```python
from build123d import *

# Parameters (mm, degrees)
SKETCH_1_R      = 1.6
EXTRUDE_1_DEPTH = 2
FILLET_1_R      = 2


with BuildPart() as part:
    # 草图1 → 凸台-拉伸1 (new body)
    with BuildSketch(Plane(origin=(0, 0, 0), x_dir=(1, 0, 0), z_dir=(0, 1, 0))):
        with BuildLine():
            Line((-130, -81.5), (130, -81.5))
            Line((130, -81.5), (130, 81.5))
            Line((130, 81.5), (90, 81.5))
            ThreePointArc((90, 81.5), (0, -8.5), (-90, 81.5))
            Line((-90, 81.5), (-130, 81.5))
            Line((-130, 81.5), (-130, -81.5))
        make_face()
        with Locations(Location((-122, -33.5, 0), (0, 0, 270))):
            Circle(SKETCH_1_R, mode=Mode.SUBTRACT)
        with Locations(Location((-122, -13.5, 0), (0, 0, 270))):
            Circle(SKETCH_1_R, mode=Mode.SUBTRACT)
        with Locations(Location((-122, 36.5, 0), (0, 0, 270))):
            Circle(SKETCH_1_R, mode=Mode.SUBTRACT)
        with Locations(Location((-82.27241336, 34, 0), (0, 0, 270))):
            Circle(SKETCH_1_R, mode=Mode.SUBTRACT)
        with Locations(Location((-47.5, -0.77241336, 0), (0, 0, 270))):
            Circle(SKETCH_1_R, mode=Mode.SUBTRACT)
        with Locations(Location((122, -33.5, 0), (0, 0, 270))):
            Circle(SKETCH_1_R, mode=Mode.SUBTRACT)
        with Locations(Location((0, -13.5, 0), (0, 0, 270))):
            Circle(SKETCH_1_R, mode=Mode.SUBTRACT)
        with Locations(Location((47.5, -0.77241336, 0), (0, 0, 270))):
            Circle(SKETCH_1_R, mode=Mode.SUBTRACT)
        with Locations(Location((122, -13.5, 0), (0, 0, 270))):
            Circle(SKETCH_1_R, mode=Mode.SUBTRACT)
        with Locations(Location((82.27241336, 34, 0), (0, 0, 270))):
            Circle(SKETCH_1_R, mode=Mode.SUBTRACT)
        with Locations(Location((122, 36.5, 0), (0, 0, 270))):
            Circle(SKETCH_1_R, mode=Mode.SUBTRACT)
        with Locations(Location((-122, 56.5, 0), (0, 0, 270))):
            Circle(SKETCH_1_R, mode=Mode.SUBTRACT)
        with Locations(Location((122, 56.5, 0), (0, 0, 270))):
            Circle(SKETCH_1_R, mode=Mode.SUBTRACT)
    extrude(amount=EXTRUDE_1_DEPTH)

    # 圆角1
    fillet_1_edges = [part.edges().sort_by_distance(p)[0] for p in [
        (90, 1, -81.5),
        (130, 1, -81.5),
        (130, 1, 81.5),
        (-130, 1, 81.5),
        (-130, 1, -81.5),
        (-90, 1, -81.5),
    ]]
    fillet(fillet_1_edges, radius=FILLET_1_R)


solid = part.part
```
Source: CAD feature listing. Evaluate the final solid. Frame: model axes, mm. Round coordinates to 2 decimals unless told otherwise and drop trailing zeros. Loops run counter-clockwise (first coordinate to the right, second up) from the corner with the lowest first, then second, coordinate; pieces in that order, holes last.
1. Section query D-D on x = 9. Output: boundary loops of the cut face in (y, z), and give its area (3 significant figures).
2. Section query A-A on z = -48. Output: boundary loops of the cut face in (x, y), and give its area (3 significant figures).
3. Mould query, pull axis X, two halves, no side actions, for faces 1 (the flat face through (-2, 0, 17)), 2 (the cylindrical face through (1.95, 0.99, 8.48)). Classes: released by +X, released by -X, zero draft, split by the parting line, or undercut.
4. Section query B-B on y = 1.55. Give the number of separate pieces and of enclosed holes in the cut face, and give its area (3 significant figures).
5. Section query C-C on z = -71. Output: boundary loops of the cut face in (x, y), and give its area (3 significant figures).
6. Ray query, L1, parallel to Z at x = -122, y = 0.5; L2, parallel to X at y = 1.3, z = 13.5; L3, parallel to X at y = 1.5, z = 33.5. Return the intervals inside material, ascending.
7. Contact query for a flat-ended pin moving along its axis: pin 1 (1.9 mm diameter, centred on x = -122, z = 13.5, fed in from +Y). Output: stop coordinate, or through.
Answers below:
1. outline: (0, 8.05) - (2, 8.05) - (2, 81.5) - (0, 81.5) - close
1. area: 147 mm2
2. outline: (-130, 0) - (-83.53, 0) - (-83.53, 2) - (-130, 2) - close; (83.53, 0) - (130, 0) - (130, 2) - (83.53, 2) - close
2. area: 186 mm2
3. face 1: zero draft
3. face 2: undercut
4. separate pieces: 1
4. enclosed holes: 13
4. area: 29,500 mm2
5. outline: (-130, 0) - (-89.39, 0) - (-89.39, 2) - (-130, 2) - close; (89.39, 0) - (130, 0) - (130, 2) - (89.39, 2) - close
5. area: 162 mm2
6. L1: z = -81.5 to -58.1, -54.9 to -38.1, -34.9 to 11.9, 15.1 to 31.9, 35.1 to 81.5
6. L2: x = -130 to -123.6, -120.4 to -1.6, 1.6 to 120.4, 123.6 to 130
6. L3: x = -130 to -123.6, -120.4 to 120.4, 123.6 to 130
7. pin 1: passes through
